Read the model definition and answer for the solid it produces. Units are mm, in the model's axes. A direction names the side the tool comes from. Coordinates: 2 decimals unless noted, no trailing zeros. Order: outer loops, then holes, each group sorted by start corner. A loop starts at its lowest first (then second) coordinate and runs counter-clockwise, first axis right, second up. Notation, with made-up numbers: M 4,40.25 L 11,40.25 A14 cw 11,44.25 Z; hole C -30.5,19.25 d1. An arc over 180 degrees is marked long. Write each question's results on one line, items separated by ' | '.
```python
from build123d import *

# Parameters (mm, degrees)
SKETCH_1_R      = 75
EXTRUDE_1_DEPTH = 100
SKETCH_2_R      = 10
EXTRUDE_2_DEPTH = 100
FILLET_1_R      = 5


with BuildPart() as part:
    # 草图1 → 凸台-拉伸1 (new body)
    with BuildSketch(Plane.XY):
        Circle(SKETCH_1_R)
    extrude(amount=EXTRUDE_1_DEPTH)

    # 草图2 → 凸台-拉伸2 (add)
    with BuildSketch(Plane.XY.offset(100)):
        Circle(SKETCH_2_R)
    extrude(amount=EXTRUDE_2_DEPTH)

    # 圆角1
    fillet_1_edges = [part.edges().sort_by_distance(p)[0] for p in [
        (-10, 0, 100),
    ]]
    fillet(fillet_1_edges, radius=FILLET_1_R)


solid = part.part
```
(1) The part is cut by section D-D, the plane x = -21. Write down the section's boundary in (y, z).
Conclusion:
outline: M -72,0 L 72,0 L 72,100 L -72,100 Z
(2) The part is cut by section C-C, the plane z = 133. Write down the section's boundary in (x, y).
Conclusion:
outline: C 0,0 d20
(3) Given pin 1 (2 mm diameter, centred on y = 34.5, z = 43.5, fed in from +X); pin 2 (5 mm diameter, centred on x = 0, z = 110.5, fed in from +Y); pin 3 (1.5 mm diameter, centred on x = 54, y = 18, fed in from +Z), each flat-ended and moving along its own axis, determine where each tip first touches the part or whether it passes through.
Conclusion:
pin 1: x = 67.1 | pin 2: y = 10 | pin 3: z = 100
(4) Straight lines are drawn through the part: line 1 (Z direction, x = -51, y = -34.5); line 2 (X direction, y = 22.5, z = 98); line 3 (Y direction, x = -46.5, z = 18.5). For each, find the intervals that lie inside material, in ascending order.
Conclusion:
line 1: 0 to 100 | line 2: -71.55 to 71.55 | line 3: -58.85 to 58.85
(5) For faces 1 (the cylindrical face through (-2.17, -9.76, 151.84)), 2 (the flat face through (-1, 1, 0)), determine the directions among +Z, -Z, +X, -X, +Y, -Y from which every point of the face is accessible in a straight line to the end or side of a thin tool.
Conclusion:
face 1: +Z | face 2: -Z, +X, -X, +Y, -Y
(6) The part is cut by section A-A, the plane y = 0. Write down the section's boundary in (x, z).
Conclusion:
outline: M -75,0 L 75,0 L 75,100 L 15,100 A5 cw 10,105 L 10,200 L -10,200 L -10,105 A5 cw -15,100 L -75,100 Z
